Autodesk Inventor part; units mm, degrees
ref_plane "YZ Plane" through (0, 0, 0) normal (1, 0, 0) x (0, 1, 0)
ref_plane "XZ Plane" through (0, 0, 0) normal (0, 1, 0) x (-1, 0, 0)
ref_plane "XY Plane" through (0, 0, 0) normal (0, 0, 1) x (1, 0, 0)
sketch "Sketch1" plane through (0, 0, 0) normal (0, 1, 0) x (-1, 0, 0)
  line L0 (0, 0) -> (177.8, 0)
  line L1 (177.8, -177.8) -> (0, -177.8)
  line L2 (0, -177.8) -> (0, 0)
  line L3 (177.8, 0) -> (177.8, -82.55)
  line L4 (177.8, -82.55) -> (215.9, -82.55)
  line L5 (215.9, -82.55) -> (215.9, -95.25)
  line L6 (215.9, -95.25) -> (177.8, -95.25)
  line L7 (177.8, -95.25) -> (177.8, -177.8)
  line L8 (0, 0) -> (0, -88.9)
  line L9 (63.5, -88.9) -> (63.5, -95.25)
  line L10 (12.7, -88.9) -> (12.7, -95.25)
  line L11 (12.7, -95.25) -> (63.5, -95.25)
  line L12 (12.7, -95.25) -> (12.7, -82.55)
  line L13 (12.7, -82.55) -> (63.5, -82.55)
  line L14 (63.5, -82.55) -> (63.5, -95.25)
  dimension "d0" = 177.8
  dimension "d1" = 177.8
  dimension "d39" = 82.55
  dimension "d41" = 12.7
  dimension "d44" = 6.35
  dimension "d45" = 12.7
extrude "Extrusion1" add sketch "Sketch1" along normal blind 1.5875
sketch "Sketch2" plane through (0, 1.5875, 0) normal (0, 1, 0) x (1, 0, 0)
  line L0 (-177.8, 177.8) -> (-177.8, 0)
  line L1 (-177.8, 177.8) -> (-177.8, 165.1)
  line L2 (-177.8, 165.1) -> (-165.1, 177.8)
  line L3 (0, 177.8) -> (-177.8, 177.8)
  line L4 (-177.8, 177.8) -> (-171.45, 171.45)
  line L5 (-171.45, 171.45) -> (-158.75, 171.45)
  line L6 (-177.8, 0) -> (-165.1, 0)
  line L7 (-177.8, 0) -> (0, 0)
  line L8 (0, 177.8) -> (-12.7, 177.8)
  line L9 (0, 0) -> (0, 177.8)
  line L10 (0, 0) -> (0, 12.7)
  line L11 (0, 12.7) -> (-12.7, 0)
  line L12 (0, 0) -> (-6.35, 6.35)
  line L13 (-6.35, 6.35) -> (-6.35, 19.05)
  line L14 (-6.35, 19.05) -> (-19.05, 19.05)
  line L15 (-19.05, 19.05) -> (-31.75, 19.05)
  line L16 (-12.7, 177.8) -> (0, 165.1)
  line L17 (0, 177.8) -> (-6.35, 171.45)
  line L18 (-165.1, 0) -> (-177.8, 12.7)
  line L19 (-177.8, 0) -> (-171.45, 6.35)
  line L20 (-171.45, 6.35) -> (-171.45, 19.05)
  line L21 (-171.45, 6.35) -> (-158.75, 6.35)
  line L22 (-6.35, 171.45) -> (-6.35, 169.799)
  line L23 (-6.35, 169.799) -> (-4.699, 169.799)
  line L24 (-215.9, 82.55) -> (-177.8, 82.55)
  line L25 (-215.9, 82.55) -> (-203.2, 95.25)
  line L26 (-177.8, 95.25) -> (-215.9, 95.25)
  line L27 (-215.9, 82.55) -> (-197.9395, 82.55) construction
  line L28 (-203.2, 95.25) -> (-215.9, 95.25)
  line L29 (-215.9, 95.25) -> (-203.2, 82.55)
  point P0 (-209.55, 88.9)
  dimension "d4" = 12.7
  dimension "d5" = 45
  dimension "d6" = 12.7
  dimension "d7" = 12.7
  dimension "d12" = 12.7
  dimension "d28" = 1.651
  dimension "d42" = 45
hole "Hole2" at (-171.45, 1.5875, -171.45) at (-158.75, 1.5875, -171.45) at (-19.05, 1.5875, -19.05) at (-31.75, 1.5875, -19.05) at (-171.45, 1.5875, -19.05) at (-158.75, 1.5875, -6.35) at (-4.699, 1.5875, -169.799) at (-209.55, 1.5875, -88.9) direction (0, -1, 0) diameter 4.7625 end through all
sketch "Sketch3" plane through (0, 1.5875, 0) normal (0, 1, 0) x (1, 0, 0)
  line L0 (0, 0) -> (0, 12.7)
  line L1 (0, 0) -> (0, 177.8)
  line L2 (0, 12.7) -> (-12.7, 0)
  line L3 (-177.8, 0) -> (0, 0)
  line L4 (-12.7, 0) -> (0, 0)
  line L5 (0, 0) -> (-6.35, 6.35)
  line L6 (-6.35, 6.35) -> (-82.55, 6.35)
  dimension "d29" = 12.7
  dimension "d30" = 45
  dimension "d31" = 76.2
hole "Hole3" at (-82.55, 1.5875, -6.35) direction (0, -1, 0) diameter 4.7625 end through all
properties part number "shoot" material "ABS Plastic"
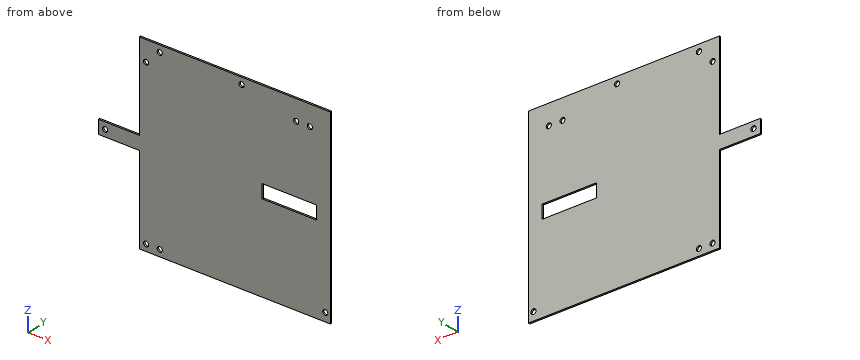
Source: CAD feature listing. Evaluate the final solid. Frame: model axes, mm. Give positions to 0.01 mm unless a question says otherwise; leave off trailing zeros. Write each loop counter-clockwise with the first axis right and the second up, starting at its lowest first coordinate (ties: lowest second). Pieces come first, ordered by that corner, then holes. Notation, with made-up numbers: (55, 75) -> (81, 75) arc R11 ccw to (81, 79) -> close; hole circle Ø7 at (4.5, 79). An arc over 180 degrees is marked (long way). Return JSON: item names as keys, results as strings. Group by question number.
1. Section A-A, the plane z = -88.9. Output: boundary loops of the cut face in (x, y).
2. Section B-B, the plane x = -31.75. Output: boundary loops of the cut face in (y, z), then the cut area to 3 significant figures.
3. Section C-C, the plane x = -82.55. Output: boundary loops of the cut face in (y, z).
4. Section D-D, the plane z = -19.05. Output: boundary loops of the cut face in (x, y), then the cut area to 3 significant figures.
5. Material intervals for line 1 (Z direction, x = -158.75, y = 1.1); line 2 (X direction, y = 0.7, z = -6.35); line 3 (Z direction, x = -171.45, y = 1), sorted ascending. Write a range as from..to.
6. Pin query (flat end, axial travel): pin 1 Ø0.8 at (x, y) = (-187.5, 1) entering from -Z; pin 2 Ø7.5 at (x, z) = (-209.55, -88.9) entering from +Y; pin 3 Ø0.8 at (x, y) = (-200.5, 0.5) entering from +Z; pin 4 Ø4.5 at (x, z) = (-31.75, -19.05) entering from -Y. Return the tip coordinate at first contact, or that it passes through.
Determined:
{
 "1": {"outline": "(-215.9, 0) -> (-211.93, 0) -> (-211.93, 1.59) -> (-215.9, 1.59) -> close; (-207.17, 0) -> (-63.5, 0) -> (-63.5, 1.59) -> (-207.17, 1.59) -> close; (-12.7, 0) -> (0, 0) -> (0, 1.59) -> (-12.7, 1.59) -> close"},
 "2": {"outline": "(0, -177.8) -> (1.59, -177.8) -> (1.59, -95.25) -> (0, -95.25) -> close; (0, -82.55) -> (1.59, -82.55) -> (1.59, -21.43) -> (0, -21.43) -> close; (0, -16.67) -> (1.59, -16.67) -> (1.59, 0) -> (0, 0) -> close", "area": "255 mm2"},
 "3": {"outline": "(0, -177.8) -> (1.59, -177.8) -> (1.59, -8.73) -> (0, -8.73) -> close; (0, -3.97) -> (1.59, -3.97) -> (1.59, 0) -> (0, 0) -> close"},
 "4": {"outline": "(-177.8, 0) -> (-173.83, 0) -> (-173.83, 1.59) -> (-177.8, 1.59) -> close; (-169.07, 0) -> (-34.13, 0) -> (-34.13, 1.59) -> (-169.07, 1.59) -> close; (-29.37, 0) -> (-21.43, 0) -> (-21.43, 1.59) -> (-29.37, 1.59) -> close; (-16.67, 0) -> (0, 0) -> (0, 1.59) -> (-16.67, 1.59) -> close", "area": "260 mm2"},
 "5": {"line 1": "z = -177.8..-173.83, -169.07..-8.73, -3.97..0", "line 2": "x = -177.8..-161.13, -156.37..-84.93, -80.17..0", "line 3": "z = -177.8..-173.83, -169.07..-21.43, -16.67..0"},
 "6": {"pin 1": "stops at z = -95.25", "pin 2": "stops at y = 1.59", "pin 3": "stops at z = -82.55", "pin 4": "passes through"}
}
